Geometry check sheet. Reference: the model listing, model coordinates, mm. A direction names the side the tool comes from. Round coordinates to 2 decimals unless told otherwise and drop trailing zeros. Order: outer loops, then holes, each group sorted by start corner. A loop starts at its lowest first (then second) coordinate and runs counter-clockwise, first axis right, second up. Notation, with made-up numbers: M 33,51 L 66,51 A25 cw 66,89 Z; hole C 84,14 d3. An arc over 180 degrees is marked long. Answer as a JSON object with one key per item and string values. Group by question number.
```python
from build123d import *

# Parameters (mm, degrees)
F0_R     = 1.5
F1_DEPTH = 10
F2_R     = 3
F2_R_2   = 1.5
F3_DEPTH = 3
F4_W     = 1.5
F4_H     = 1
F4_W_2   = 1
F4_H_2   = 1.5
F5_DEPTH = 2


# Not quite as in the source:
# - a fillet or chamfer that OpenCascade refuses, or shapes differently, is made with other operations: its cross-section is extruded or revolved along the edge and cut away or added


with BuildPart() as f1:
    # F0 (on Top) → F1 (new body)
    with BuildSketch(Plane.XY):
        Circle(F0_R)
    extrude(amount=-F1_DEPTH)

    # F2 (on face) → F3 (join)
    with BuildSketch(Plane.XY):
        Circle(F2_R)
        Circle(F2_R_2, mode=Mode.SUBTRACT)
        Circle(F2_R_2)
    extrude(amount=F3_DEPTH)

    # F4 (on face) → F5 (cut)
    with BuildSketch(Plane.XY.offset(3)):
        with Locations((-1.25, 0)):
            Rectangle(F4_W, F4_H)
        with Locations((0, 1.25)):
            Rectangle(F4_W_2, F4_H_2)
        Rectangle(F4_W_2, F4_H)
        with Locations((1.25, 0)):
            Rectangle(F4_W, F4_H)
        with Locations((0, -1.25)):
            Rectangle(F4_W_2, F4_H_2)
    extrude(amount=-F5_DEPTH, mode=Mode.SUBTRACT)

    # F6: fillet of radius 2 on 1 edges, made by hand

    # F6_s1 → F6_t2 (revolve, cut)
    with BuildSketch(Plane.XZ):
        with BuildLine():
            ThreePointArc((3, 1), (2.4142135624, 2.4142135624), (1, 3))
            Line((1, 3), (3, 3))
            Line((3, 3), (3, 1))
        make_face()
    revolve(axis=Axis((0, 0, 3), (0, 0, 1)), mode=Mode.SUBTRACT)


solid = f1.part
```
1) Sectioned sample at A-A (z = 0.75). Record the boundary of the cut face in (x, y), then the cut area to 3 significant figures.
2) Sectioned sample at B-B (z = -7.5). Record the boundary of the cut face in (x, y), then the cut area to 3 significant figures.
3) Go/stop test with flat-tipped pins: P1, Ø1.2, axis at y = -1.5, z = 2, coming from the -X side; P2, Ø0.5, axis at y = 0, z = 2, coming from the +X side; P3, Ø1.2, axis at x = -1, z = 2, coming from the -Y side; P4, Ø2, axis at x = 1, y = -1, coming from the +Z side. Record where each tip stops, or that it passes through.
4) Release check for a two-part mould opening along X. For faces 1 (the flat face through (0, 0, -10)), 2 (the cylindrical face through (-1.5, 0.07, -4.93)), 3 (the flat face through (0.5, -1, 2)) record: +X half, -X half, draft (parallel to the pull), parting line (faces both ways), or undercut.
5) Thickness scan on line 1 along Z through (x, y) = (0.5, 0.25); line 2 along Y through (x, z) = (1, 1.25); line 3 along Y through (x, z) = (0, 1.75). Record the ranges inside material, lowest first. Write a range as [from, to].
6) Set-up check for faces 4 (the flat face through (-1, -0.5, 2)), 5 (the cylindrical face through (-3, 0.1, 0.5)), 6 (the flat face through (1.3, -1.3, 0)): record each of +Z, -Z, +X, -X, +Y, -Y from which the full face is reachable in a straight line by a thin tool's end or side.
Final values:
{
 "1": {"outline": "C 0,0 d6", "area": "28.3 mm^2"},
 "2": {"outline": "C 0,0 d3", "area": "7.07 mm^2"},
 "3": {"P1": "stops at x = -2.71", "P2": "stops at x = 2.85", "P3": "stops at y = -2.86", "P4": "stops at z = 3"},
 "4": {"face 1": "draft", "face 2": "parting line", "face 3": "undercut"},
 "5": {"line 1": "z = [-10, 1]", "line 2": "y = [-2.81, -0.5], [0.5, 2.81]", "line 3": "y = [-2.85, -2], [2, 2.85]"},
 "6": {"face 4": "+Z", "face 5": "+Z, -Z", "face 6": "-Z"}
}
